Study the drawing (mm; zero at the part's minimum x, y, z) and answer. A direction names the side the tool comes from. Coordinates: 2 decimals unless noted, no trailing zeros. Loops run counter-clockwise (first coordinate to the right, second up) from the corner with the lowest first, then second, coordinate; pieces in that order, holes last.
Q1. Section D-D (y = 5.5) is taken. Give the vertices of the cut face in (x, z).
Q2. Section B-B (y = 1.25) is taken. Give the vertices of the cut face in (x, z).
Q3. Flat-ended cylindrical pins translate along their axes: P1, Ø4, axis at x = 12.56, z = 2.5, coming from the -Y side; P2, Ø1.4, axis at x = 2, y = 4, coming from the -Z side; P3, Ø0.5, axis at x = 2, z = 6.5, coming from the +Y side. Find the tip coordinate at first contact, or state that the pin passes through.
Q4. Section A-A (z = 2.5) is taken. Give the vertices of the cut face in (x, y).
Q5. Straight lines are drawn through the part: line 1 (Z direction, x = 22.75, y = 4); line 2 (Y direction, x = 22.25, z = 5.45); line 3 (Y direction, x = 23.25, z = 2.5). For each, find the intervals that lie inside material, in ascending order.
Q6. Section C-C (x = 2.75) is taken. Give the vertices of the cut face in (y, z).
Q7. Which of the six approach directions +Z, -Z, +X, -X, +Y, -Y give full straight-line access (tool end or side, diameter ignored) to the marked faces 1, 2 and 3?
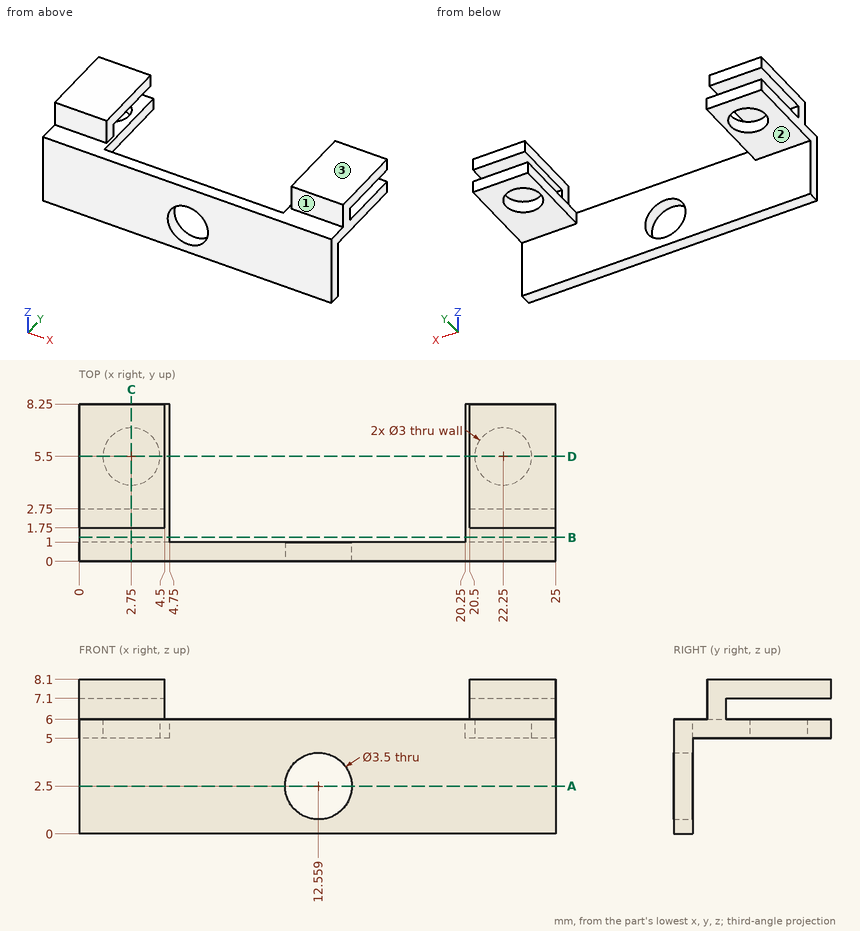
Numbers:
1. outline: (0, 5) - (1.25, 5) - (1.25, 6) - (0, 6) - close; (0, 7.1) - (4.5, 7.1) - (4.5, 8.1) - (0, 8.1) - close; (4.25, 5) - (4.75, 5) - (4.75, 6) - (4.25, 6) - close; (20.25, 5) - (20.75, 5) - (20.75, 6) - (20.25, 6) - close; (20.5, 7.1) - (25, 7.1) - (25, 8.1) - (20.5, 8.1) - close; (23.75, 5) - (25, 5) - (25, 6) - (23.75, 6) - close
2. outline: (0, 5) - (4.75, 5) - (4.75, 6) - (0, 6) - close; (20.25, 5) - (25, 5) - (25, 6) - (20.25, 6) - close
3. P1: stops at y = 0
3. P2: stops at z = 5
3. P3: stops at y = 2.75
4. outline: (0, 0) - (10.81, 0) - (10.81, 1) - (0, 1) - close; (14.31, 0) - (25, 0) - (25, 1) - (14.31, 1) - close
5. line 1: z = 5 to 6, 7.1 to 8.1
5. line 2: y = 0 to 4, 7 to 8.25
5. line 3: y = 0 to 1
6. outline: (0, 0) - (1, 0) - (1, 5) - (4, 5) - (4, 6) - (2.75, 6) - (2.75, 7.1) - (8.25, 7.1) - (8.25, 8.1) - (1.75, 8.1) - (1.75, 6) - (0, 6) - close; (7, 5) - (8.25, 5) - (8.25, 6) - (7, 6) - close
7. face 1: +Z, +X, -X, -Y
7. face 2: -Z, +X, -X, +Y
7. face 3: +Z, +X, -X, +Y, -Y
